from build123d import *

# Parameters (mm, degrees)
SKETCH1_R            = 34
SKETCH1_R_2          = 18
BOSS_EXTRUDE1_DEPTH  = 22.5
SKETCH2_R            = 16
SKETCH2_R_2          = 8
BOSS_EXTRUDE2_DEPTH  = 22.5
BOSS_EXTRUDE4_DEPTH  = 7.5
BOSS_EXTRUDE5_DEPTH  = 7.5
BOSS_EXTRUDE13_DEPTH = 12.5
BOSS_EXTRUDE14_DEPTH = 7.5
FILLET14_R           = 10
FILLET16_R           = 8
FILLET17_R           = 8


with BuildPart() as part:
    # Sketch1 → Boss-Extrude1 (new, symmetric)
    with BuildSketch(Plane.XY):
        with Locations(Location((0, 0, 0), (0, 0, 180))):
            Circle(SKETCH1_R)
        with Locations(Location((0, 0, 0), (0, 0, 180))):
            Circle(SKETCH1_R_2, mode=Mode.SUBTRACT)
    extrude(amount=BOSS_EXTRUDE1_DEPTH, both=True)



with BuildPart() as body_2:
    # Sketch2 → Boss-Extrude2 (new, symmetric)
    with BuildSketch(Plane.XY):
        with Locations(Location((97, -28, 0), (0, 0, 180))):
            Circle(SKETCH2_R)
        with Locations(Location((97, -28, 0), (0, 0, 180))):
            Circle(SKETCH2_R_2, mode=Mode.SUBTRACT)
    extrude(amount=BOSS_EXTRUDE2_DEPTH, both=True)


with BuildPart() as part_1:
    add(part.part)

    add(body_2.part)  # Boss-Extrude4 merges body 2
    # Sketch4 → Boss-Extrude4 (add, symmetric)
    with BuildSketch(Plane.XY):
        with BuildLine():
            ThreePointArc((33.206005609, -7.1003724), (51.777283235, -34.98924979), (82.412015856, -21.417404229))
            ThreePointArc((82.412015856, -21.417404229), (81.371091146, -25.082275632), (81.074017469, -28.880505994))
            ThreePointArc((81.074017469, -28.880505994), (51.369473654, -37.991410417), (30.470988374, -14.999633287))
            ThreePointArc((30.470988374, -14.999633287), (32.120493939, -11.147640651), (33.206005609, -7.1003724))
        make_face()
    extrude(amount=BOSS_EXTRUDE4_DEPTH, both=True)

    # Sketch5 → Boss-Extrude5 (add, symmetric)
    with BuildSketch(Plane.XY):
        with BuildLine():
            ThreePointArc((-34.031526001, -0.792277944), (25.431977893, -71.913257024), (110.881269035, -35.961614448))
            ThreePointArc((110.881269035, -35.961614448), (107.27285681, -40.164612784), (102.451649001, -42.892577053))
            ThreePointArc((102.451649001, -42.892577053), (30.885190637, -69.988396494), (-27.207046107, -20.176415768))
            ThreePointArc((-27.207046107, -20.176415768), (-31.977671369, -10.96258702), (-34.031526001, -0.792277944))
        make_face()
    extrude(amount=BOSS_EXTRUDE5_DEPTH, both=True)



with BuildPart() as body_2_2:
    # Sketch8 → Boss-Extrude13 (new, symmetric)
    with BuildSketch(Plane.XY):
        with BuildLine():
            ThreePointArc((-14.937494573, 90.972331385), (-50.475974734, 50.279724458), (-65.522765853, -1.609252288))
            ThreePointArc((-65.522765853, -1.609252288), (-92.080170519, -24.948152378), (-115.419070609, 1.609252288))
            ThreePointArc((-115.419070609, 1.609252288), (-94.353563042, 74.253819732), (-44.599690817, 131.223469431))
            ThreePointArc((-44.599690817, 131.223469431), (-9.643023672, 125.92899853), (-14.937494573, 90.972331385))
        make_face()
        with BuildLine():
            ThreePointArc((-104.441883562, 0.901181281), (-91.372099512, -13.970965332), (-76.499952899, -0.901181281))
            ThreePointArc((-76.499952899, -0.901181281), (-60.129044162, 55.554025418), (-21.463177747, 99.827581755))
            ThreePointArc((-21.463177747, 99.827581755), (-18.498274042, 119.403315356), (-38.074007643, 122.368219061))
            ThreePointArc((-38.074007643, 122.368219061), (-84.700493614, 68.979518772), (-104.441883562, 0.901181281))
        make_face(mode=Mode.SUBTRACT)
    extrude(amount=BOSS_EXTRUDE13_DEPTH, both=True)


with BuildPart() as part_2:
    add(part_1.part)

    add(body_2_2.part)  # Boss-Extrude14 merges body 2 2
    # Sketch8<9> → Boss-Extrude14 (add, symmetric)
    with BuildSketch(Plane.XY):
        with BuildLine():
            ThreePointArc((-4.924235101, 108.312600467), (-0.101365505, 63.440523319), (23.275646022, 24.836395161))
            ThreePointArc((23.275646022, 24.836395161), (18.02581673, 28.582349539), (12.304584847, 31.558989848))
            ThreePointArc((12.304584847, 31.558989848), (-3.899104901, 62.184418871), (-9.571104645, 96.364894046))
            ThreePointArc((-9.571104645, 96.364894046), (-6.468831174, 102.035830387), (-4.924235101, 108.312600467))
        make_face()
        with BuildLine():
            ThreePointArc((-31.919461404, -14.075384629), (-51.826123505, -6.018423189), (-71.003100626, -15.684517133))
            ThreePointArc((-71.003100626, -15.684517133), (-68.148351126, -11.256242618), (-66.285052548, -6.32802506))
            ThreePointArc((-66.285052548, -6.32802506), (-49.617118255, -2.018061944), (-33.32443821, -7.580830374))
            ThreePointArc((-33.32443821, -7.580830374), (-32.713889809, -10.847997022), (-31.919461404, -14.075384629))
        make_face()
    extrude(amount=BOSS_EXTRUDE14_DEPTH, both=True)

    # Fillet14
    # the kernel refuses this fillet: 10 mm, written as the material it adds along each edge
    with BuildSketch(Plane(origin=(-9.571104645, 96.364894046, -7.5), x_dir=(-0.7492882116327264, -0.6622440455815594, 0), z_dir=(0, 0, 1))) as fillet14_piece_1:
        with BuildLine():
            CenterArc((19.69565471, 9.999601125), FILLET14_R, 148.729139323, 121.782610057)
            Line((11.148425358, 15.19044599), (10.293702423, 15.709530477))
            ThreePointArc((10.293702423, 15.709530477), (5.099940987, 7.943295893), (-0.751496774, 0.659736764))
            Line((-0.751496774, 0.659736764), (0.215075759, -0.976597367))
            ThreePointArc((0.215075759, -0.976597367), (7.503554375, -0.509342466), (19.793902231, -0.999960113))
            Line((19.793902231, -0.999960113), (19.784970638, 0))
        make_face()
    extrude(amount=15)
    with BuildSketch(Plane(origin=(12.159345053, 31.751383086, -7.5), x_dir=(-0.5285784325634836, 0.8488844683634699, 0), z_dir=(0, 0, 1))) as fillet14_piece_2:
        with BuildLine():
            CenterArc((19.996455315, 9.960779633), FILLET14_R, 157.06784833, 107.855989322)
            ThreePointArc((10.786786288, 13.857187776), (6.303465021, 6.220170866), (0, 0))
            ThreePointArc((0, 0), (9.555828204, 0.423579966), (19.111656407, 0))
        make_face()
    extrude(amount=15)
    with BuildSketch(Plane(origin=(-32.126211784, -13.860546046, -7.5), x_dir=(-0.7488822965541873, 0.6627030299521243, 0), z_dir=(0, 0, 1))) as fillet14_piece_3:
        with BuildLine():
            CenterArc((3.122942969, 9.972317771), FILLET14_R, 236.75546449, 37.508743658)
            ThreePointArc((-2.359191707, 1.608933325), (-1.172232304, 0.815263894), (0, 0))
            ThreePointArc((0, 0), (1.933250409, -0.071973796), (3.866500819, 0))
        make_face()
    extrude(amount=15)
    with BuildSketch(Plane(origin=(-33.32443821, -7.580830374, -7.5), x_dir=(-0.9057047717229613, 0.42390903089962434, 0), z_dir=(0, 0, 1))) as fillet14_piece_4:
        with BuildLine():
            CenterArc((12.689549677, -9.834316561), FILLET14_R, 100.444283177, 56.0673219)
            ThreePointArc((3.518141468, -5.84868343), (1.823073957, -2.885842043), (0, 0))
            ThreePointArc((0, 0), (5.438378433, -0.497050317), (10.876756866, 0))
        make_face()
    extrude(amount=15)
    with BuildSketch(Plane(origin=(-66.285052548, -6.32802506, -7.5), x_dir=(0.12382892083322194, 0.9923035817557446, 0), z_dir=(0, 0, 1))) as fillet14_piece_5:
        with BuildLine():
            CenterArc((15.518466833, -9.995933117), FILLET14_R, 88.36588285, 104.037213694)
            Line((5.751860117, -12.143814227), (4.775199446, -12.358602338))
            ThreePointArc((4.775199446, -12.358602338), (2.660832169, -6.173787211), (-0.784932001, -0.619581919))
            Line((-0.784932001, -0.619581919), (0.131376491, 0.991332546))
            ThreePointArc((0.131376491, 0.991332546), (4.717150823, 0.82611724), (15.832152273, 0.999593312))
            Line((15.832152273, 0.999593312), (15.803635414, 0))
        make_face()
    extrude(amount=15)
    # the kernel refuses this fillet: 10 mm, written as the material it takes off along each edge
    with BuildSketch(Plane(origin=(23.275646022, 24.836395161, 12.075662987), x_dir=(-0.775723763432973, 0.6310726129736459, 0), z_dir=(0, 0, -1))) as fillet14_2_piece_1:
        with BuildLine():
            CenterArc((3.231710715, -9.655465783), FILLET14_R, 98.150393055, 6.933334265)
            ThreePointArc((1.813991439, 0.243527704), (0.907531451, 0.117773287), (0, 0))
            ThreePointArc((0, 0), (0.314703895, 0.001074211), (0.62940779, 0))
        make_face()
    extrude(amount=24.151325973, mode=Mode.SUBTRACT)

    # Fillet16
    fillet16_edges = [part_2.edges().sort_by_distance(p)[0] for p in [
        (102.283564786, -43.10244825, 0),
        (-27.073199852, -20.567981178, 0),
    ]]
    fillet(fillet16_edges, radius=FILLET16_R)

    # Fillet17
    fillet17_edges = [part_2.edges().sort_by_distance(p)[0] for p in [
        (30.481870475, -15.06172541, 0),
        (81.027337873, -28.934914209, 0),
    ]]
    fillet(fillet17_edges, radius=FILLET17_R)


solid = part_2.part
Can you work these out from the model? Positions are in its coordinate system, mm. A direction names the side the tool comes from. Coordinates: 2 decimals unless noted, no trailing zeros. Write each loop counter-clockwise with the first axis right and the second up, starting at its lowest first coordinate (ties: lowest second). Pieces come first, ordered by that corner, then holes.
Q1. Imagine slicing it at B-B, the plane x = -61.5. List the corners of the cut face in (y, z) for me, plus the area to 3 significant figures.
Results found:
outline: (-8.32, -7.5) - (0.75, -7.5) - (0.75, 7.5) - (-8.32, 7.5) - close; (22.78, -12.5) - (52.98, -12.5) - (52.98, 12.5) - (22.78, 12.5) - close; (101.35, -12.5) - (117.04, -12.5) - (117.04, 12.5) - (101.35, 12.5) - close
area: 1,280 mm2
Q2. Which directions (+Z, -Z, +X, -X, +Y, -Y) give clear straight access to the entire face, cutting with the end or side of a thin tool? Please do faces 1 (the face through (-14.33, 85.24, -0.11)), 2 (the face through (109.697, -18.264, 0.315)), 3 (the face through (2, -60, 7.5)).
Results found:
face 1: +Z, -Z
face 2: none
face 3: +Z, -Y
Q3. For P1, Ø4, axis at x = -49.5, z = 8.5, coming from the -Y side; P2, Ø4, axis at y = 80, z = -7, coming from the +X side; P3, Ø12, axis at y = 62, z = -9, coming from the +X side, each with a flat end and sliding along its axis, tell me the tip position at first contact or that it passes through.
Results found:
P1: stops at y = -6.17
P2: stops at x = -3.87
P3: stops at x = 2.65
Q4. Imagine slicing it at A-A, the plane y = 56. List the corners of the cut face in (x, z) for me, plus the area to 3 significant figures.
Results found:
outline: (-103, -12.5) - (-91.07, -12.5) - (-91.07, 12.5) - (-103, 12.5) - close; (-59.88, -12.5) - (-47.15, -12.5) - (-47.15, 12.5) - (-59.88, 12.5) - close; (-1.6, -7.5) - (2.73, -7.5) - (2.73, 7.5) - (-1.6, 7.5) - close
area: 682 mm2
Q5. If we mould it in two halves opening along X, with no side actions, what happens to faces 4 (the face through (100.8, -35.3, -22.5)), 5 (the face through (51.48, -34.9, 0.11)), 6 (the face through (-0.583, 64.902, -0.105))? For each: +X half, -X half, draft (parallel to the pull), parting line (faces both ways), or undercut.
Results found:
face 4: draft
face 5: undercut
face 6: +X half
Q6. Please list where these lines run through material, in increasing order: L1, parallel to X at y = 74, z = 0; L2, parallel to Y at x = -12.5, z = 0; L3, parallel to Y at x = 97, z = -12.
Results found:
L1: x = -94.49 to -81.84, -48.01 to -33.66, -7.15 to -3.06
L2: y = -50.07 to -45.16, -38.16 to -12.95, 12.95 to 31.62, 84.37 to 129.18
L3: y = -44 to -36, -20 to -12
Q7. Imagine slicing it at C-C, the plane x = 97. List the corners of the cut face in (y, z) for me, plus the area to 3 significant figures.
Results found:
outline: (-53.18, -7.5) - (-44, -7.5) - (-44, -22.5) - (-36, -22.5) - (-36, 22.5) - (-44, 22.5) - (-44, 7.5) - (-53.18, 7.5) - close; (-20, -22.5) - (-12, -22.5) - (-12, 22.5) - (-20, 22.5) - close
area: 858 mm2
